Check sheet for the modelled part. Datum: model origin and axes. Units: mm. A direction names the side the tool comes from. Round coordinates to 2 decimals unless told otherwise and drop trailing zeros. Order: outer loops, then holes, each group sorted by start corner. A loop starts at its lowest first (then second) coordinate and runs counter-clockwise, first axis right, second up. Notation, with made-up numbers: M 77,-3.5 L 124,-3.5 A16 cw 124,16.5 Z; hole C 36.5,23.5 d7. An arc over 180 degrees is marked long. One line per item, written item: value. Start each with the question number.
(1) Cross-section at B-B, the plane x = 2.25. Enter the section's corners in (y, z).
(2) Thickness scan on L1, parallel to Z at x = 11, y = -4; L2, parallel to X at y = 1.75, z = -12; L3, parallel to Y at x = 4.5, z = -118.5. Record the ranges inside material, lowest first.
(3) Depth check by flat-ended pin: pin 1 Ø4 at (y, z) = (0, -182) entering from -X; pin 2 Ø12 at (x, z) = (3, -67.5) entering from -Y; pin 3 Ø2.5 at (y, z) = (-2, -158) entering from -X; pin 4 Ø12 at (x, z) = (-2.5, -165) entering from +Y. Enter the tip coordinate at first touch or a pass-through.
(4) Cross-section at C-C, the plane z = -198. Enter the section's corners in (x, y), and give its area (4 significant figures).
(5) Access from +Z, -Z, +X, -X, +Y, -Y to the whole of each face (thin tool, end or side, straight path). Record for faces 1 (the face through (5, -1, -254)), 2 (the face through (0, 2, -121)), 3 (the face through (7, 0, -120)).
(6) Cross-section at A-A, the plane y = -3.5. Enter the section's corners in (x, z), and give its area (3 significant figures).
Autodesk Inventor part; units mm, degrees
ref_plane "YZ Plane" through (0, 0, 0) normal (1, 0, 0) x (0, 1, 0)
ref_plane "XZ Plane" through (0, 0, 0) normal (0, 1, 0) x (-1, 0, 0)
ref_plane "XY Plane" through (0, 0, 0) normal (0, 0, 1) x (1, 0, 0)
sketch "Sketch1" plane through (0, 0, 0) normal (1, 0, 0) x (0, 1, 0)
  line L0 (0, 0) -> (3.81, 0)
  line L1 (3.81, 0) -> (3.81, -254)
  line L2 (3.81, -254) -> (0, -254)
  line L3 (0, -254) -> (0, 0)
  dimension "d0" = 254
  dimension "d1" = 3.81
extrude "Extrusion1" add sketch "Sketch1" along normal blind 15
sketch "Sketch2" plane through (0, 0, -254) normal (0, -1, 0) x (1, 0, 0)
  line L0 (15, 254) -> (15, 0)
  line L1 (0, 0) -> (0, 254)
  line L2 (15, 0) -> (0, 0)
  line L3 (0, 0) -> (0, 17.0864)
  line L4 (0, 17.0864) -> (15, 17.0864)
  line L5 (15, 17.0864) -> (15, 0)
  dimension "d4" = 17.0864
extrude "Extrusion2" add sketch "Sketch2" along normal blind 5.08
sketch "Sketch3" plane through (0, 0, 0) normal (-1, 0, 0) x (0, 0, 1)
  line L0 (-254, 3.81) -> (-254, -5.08)
  line L1 (0, 3.81) -> (-254, 3.81)
  line L2 (-254, -5.08) -> (-245.8991, -5.08)
  line L3 (-245.8991, -5.08) -> (-245.8991, 3.81)
  line L4 (-245.8991, 3.81) -> (-254, 3.81)
  line L5 (-254, 3.81) -> (-254, -5.08)
  point P0 (0, 0)
  dimension "d7" = 8.1008
extrude "Extrusion3" add sketch "Sketch3" along normal blind 5.08
properties part number "rails"
Values found:
1. outline: M -5.08,-254 L 3.81,-254 L 3.81,0 L 0,0 L 0,-236.91 L -5.08,-236.91 Z
2. L1: -254 to -236.91
2. L2: 0 to 15
2. L3: 0 to 3.81
3. pin 1: x = 0
3. pin 2: y = 0
3. pin 3: through
3. pin 4: y = 3.81
4. outline: M 0,0 L 15,0 L 15,3.81 L 0,3.81 Z
4. area: 57.15 mm^2
5. face 1: -Z, +X, -X, +Y, -Y
5. face 2: +Z, -X, +Y, -Y
5. face 3: +Z, +X, -X, -Y
6. outline: M -5.08,-254 L 15,-254 L 15,-236.91 L 0,-236.91 L 0,-245.9 L -5.08,-245.9 Z
6. area: 297 mm^2
